Part print with two shaded views. Sizes in mm from the minimum x, y, z corner. Round coordinates to 2 decimals unless told otherwise and drop trailing zeros. Loops run counter-clockwise (first coordinate to the right, second up) from the corner with the lowest first, then second, coordinate; pieces in that order, holes last. Notation, with made-up numbers: M 58.25,-19 L 99.25,-19 A21 ccw 99.25,15 Z; hole C -16.75,58 d10. An arc over 180 degrees is marked long. Put each result on its own line as item: value. Start each with the question number.
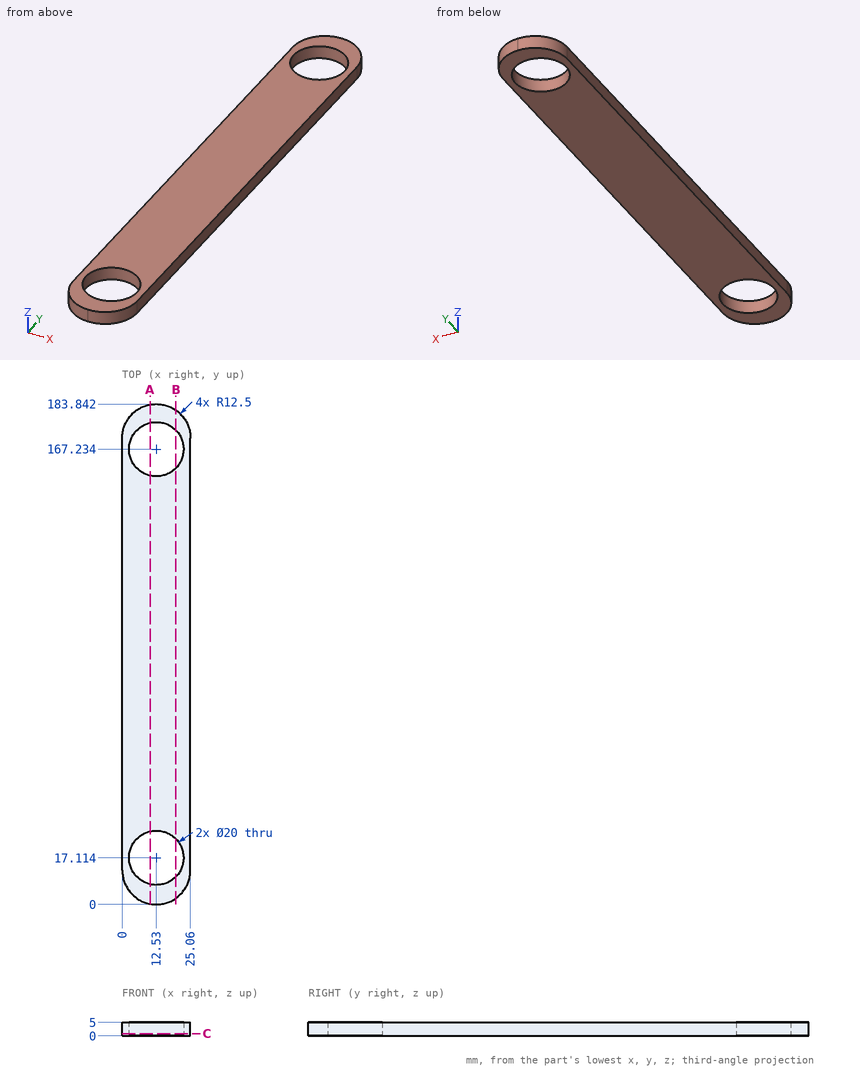
(1) Cut at A-A on x = 10.25. Count the separate pieces of the cut face and the enclosed holes in it.
(2) Cut at C-C on z = 0.9. List the corners of the cut face in (x, y).
(3) Cut at B-B on x = 19.75. List the corners of the cut face in (y, z) (1 decimal).
(4) Drill centre lines: line 1 along Y through (x, z) = (12.5, 1.4) (1 decimal); line 2 along Y through (x, z) = (4.25, 2.3) (1 decimal); line 3 along X through (y, z) = (174, 2.35) (1 decimal). Where is each one in solid material? Low to high.
Taken from the geometry:
1. separate pieces: 3
1. enclosed holes: 0
2. outline: M 0,12.5 A12.5 ccw 12.5,0 L 12.56,0 A12.5 ccw 25.06,12.5 L 25.06,171.34 A12.5 ccw 12.56,183.84 L 12.5,183.84 A12.5 ccw 0,171.34 Z; hole C 12.53,17.11 d20; hole C 12.53,167.23 d20
3. outline: M 2.3,0 L 10.2,0 L 10.2,5 L 2.3,5 Z; M 24,0 L 160.3,0 L 160.3,5 L 24,5 Z; M 174.2,0 L 181.6,0 L 181.6,5 L 174.2,5 Z
4. line 1: 0 to 7.1, 27.1 to 157.2, 177.2 to 183.8
4. line 2: 3.1 to 11.5, 22.7 to 161.6, 172.8 to 180.7
4. line 3: 0.3 to 5.2, 19.9 to 24.8
